Study the drawing (mm; zero at the part's minimum x, y, z) and answer. Round coordinates to 2 decimals unless told otherwise and drop trailing zeros. Write each loop counter-clockwise with the first axis right and the second up, starting at its lowest first coordinate (ties: lowest second). Pieces come first, ordered by that corner, then holes. Notation, with made-up numbers: (-16.5, 36) -> (19.5, 36) arc R25 cw to (19.5, 48) -> close; hole circle Ø2 at (1.5, 75). An arc over 180 degrees is marked (long way). Return JSON: item names as keys, results as strings.
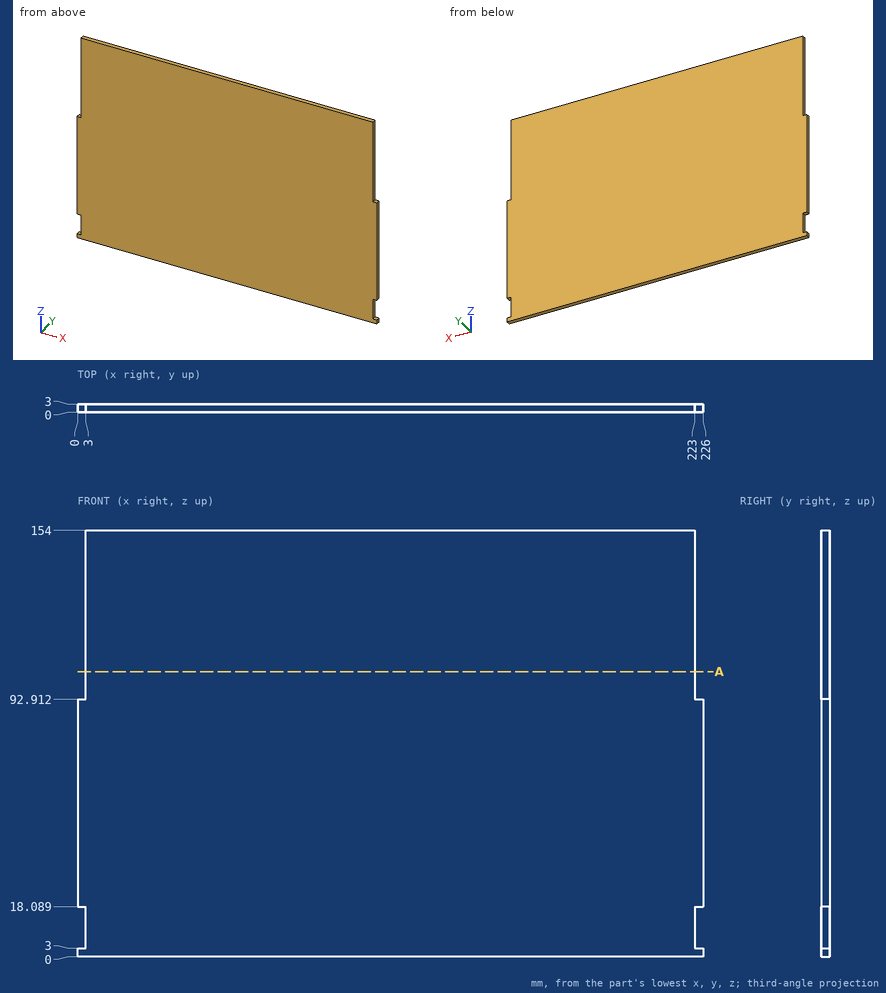
Item 1: Flat-ended cylindrical pins translate along their axes: pin 1 (1.5 mm diameter, centred on y = 1, z = 129.5, fed in from -X); pin 2 (0.9 mm diameter, centred on x = 1.5, y = 2, fed in from +Z); pin 3 (0.9 mm diameter, centred on y = 1.5, z = 7, fed in from +X). Find the tip coordinate at first contact, or state that the pin passes through.
Worked answers:
{"pin 1": "stops at x = 3", "pin 2": "stops at z = 92.91", "pin 3": "stops at x = 223"}
Item 2: A straight line is drawn through the part: L1, parallel to X at y = 0.7, z = 95.5. Find the intervals that lie inside material, in ascending order. Write a range as [from, to].
Worked answers:
{"L1": "x = [3, 223]"}
Item 3: Section A-A (z = 103) is taken. Give the vertices of the cut face in (x, y).
Worked answers:
{"outline": "(3, 0) -> (223, 0) -> (223, 3) -> (3, 3) -> close"}
